Part model, mm, in its own coordinate system. A direction names the side the tool comes from. Coordinates: 2 decimals unless noted, no trailing zeros. Loops run counter-clockwise (first coordinate to the right, second up) from the corner with the lowest first, then second, coordinate; pieces in that order, holes last. Notation, with made-up numbers: M 29.25,-30 L 82.25,-30 A7 cw 82.25,-23 Z; hole C 48.5,-15 d10. An arc over 180 degrees is marked long. Use a Markdown table: item, result. Add a question column.
1) Pull direction Y, two halves, no side cores. Call faces 1 (the flat face through (8, 0, 6.35)), 2 (the cylindrical face through (0.53, 16.36, 3.22)), 3 (the cylindrical face through (3.46, -6.016, 12.789)): released by +Y, released by -Y, zero draft, split by the parting line, or undercut.
2) Band-saw the part on B-B (y = 0). List the corners of the cut face in (x, z).
3) Band-saw the part on C-C (z = 16). List the corners of the cut face in (x, y) (1 decimal), plus the area to 3 significant figures.
4) Band-saw the part on D-D (x = 6). List the corners of the cut face in (y, z).
5) Tool access for faces 4 (the cylindrical face through (6.94, -0.01, 12.79)), 5 (the flat face through (-5.408, -3.079, 12.611)), 6 (the cylindrical face through (3.48, 6.004, 12.789)), 7 (the cylindrical face through (-6.94, 0.01, 12.79)): list every direction of +Z, -Z, +X, -X, +Y, -Y with a clear straight run to the whole face (end or side of a thin tool).
6) Wall check: probe 1 along Y at (x, z) = (0, 5.25); probe 2 along Z at (x, y) = (-8.5, 2); probe 3 along Y at (x, z) = (13.5, 4.5). Give the ranges that are in metal, low to high. Write a range as from..to.
7) Pin check, flat tips, straight feed: pin 1 Ø1.7 at (x, y) = (0, 15.08) entering from +Z; pin 2 Ø2.5 at (x, z) = (-1, 9.5) entering from +Y; pin 3 Ø10 at (y, z) = (1.5, 12) entering from -X; pin 4 Ø1 at (x, z) = (5.5, 8.5) entering from +Y. Stop position of each tip, or through.
8) Band-saw the part on A-A (x = 0). List the corners of the cut face in (y, z).
Autodesk Fusion 360 part; units mm, degrees
sketch "Sketch1" plane through (0, 0, 0) normal (0, 0, 1) x (1, 0, 0)
  circle A0 centre (0, 0) radius 18.2563
  circle A1 centre (0, 0) radius 15.0812 construction
  line L0 (0, 0) -> (0, 18.2563) construction
  line L1 (3.5929, -6.223) -> (7.1857, 0)
  line L2 (7.1857, 0) -> (3.5929, 6.223)
  line L3 (3.5929, 6.223) -> (-3.5929, 6.223)
  line L4 (-3.5929, 6.223) -> (-7.1857, 0)
  line L5 (-7.1857, 0) -> (-3.5929, -6.223)
  line L6 (-3.5929, -6.223) -> (3.5929, -6.223)
  point P0 (0, 15.0812)
  dimension "d1" = 36.5125
  dimension "d2" = 30.1625
  dimension "d3" = 6.223
extrude "Extrude1" add sketch "Sketch1" along normal blind 6.35
extrude "Extrude2" add sketch "Sketch1" along normal blind 19.05 contours L1 L2 L3 L4 L5 L6
hole "Hole1" at (0, 15.0812, 0) direction (0, 0, 1) diameter 2.7686 depth 6.35 tip angle 118
pattern_circular "C-Pattern1" count 3 over 360 about axis through (0, 0, 0) along (0, 0, 1) of "Hole1"
fillet "Fillet1" radius 1.5875 6 edges at (3.5929, -6.223, 12.7) (-3.5929, -6.223, 12.7) (-7.1857, 0, 12.7) (-3.5929, 6.223, 12.7) (3.5929, 6.223, 12.7) (7.1857, 0, 12.7)
equation "d6 = d4 + shankLength"
equation "d14 = ( 1 / 16 ) * 1 in"
equation "shankLength = 0.5 in"
Entries:
| question | item | result |
|---|---|---|
| 1 | face 1 | zero draft |
| 1 | face 2 | undercut |
| 1 | face 3 | released by -Y |
| 2 | outline | M -18.26,0 L 18.26,0 L 18.26,6.35 L 6.94,6.35 L 6.94,19.05 L -6.94,19.05 L -6.94,6.35 L -18.26,6.35 Z |
| 3 | outline | M -6.7,-0.8 L -4.1,-5.4 A1.6 ccw -2.7,-6.2 L 2.7,-6.2 A1.6 ccw 4.1,-5.4 L 6.7,-0.8 A1.6 ccw 6.7,0.8 L 4.1,5.4 A1.6 ccw 2.7,6.2 L -2.7,6.2 A1.6 ccw -4.1,5.4 L -6.7,0.8 A1.6 ccw Z |
| 3 | area | 133 mm2 |
| 4 | outline | M -17.24,0 L 17.24,0 L 17.24,6.35 L 2.05,6.35 L 2.05,19.05 L -2.05,19.05 L -2.05,6.35 L -17.24,6.35 Z |
| 5 | face 4 | +Z, +X |
| 5 | face 5 | +Z, -X, -Y |
| 5 | face 6 | +Z, +X, +Y |
| 5 | face 7 | +Z, -X |
| 6 | probe 1 | -18.26..13.7, 16.47..18.26 |
| 6 | probe 2 | 0..6.35 |
| 6 | probe 3 | -12.29..-8.85, -6.23..12.29 |
| 7 | pin 1 | through |
| 7 | pin 2 | y = 6.22 |
| 7 | pin 3 | x = -6.94 |
| 7 | pin 4 | y = 3.79 |
| 8 | outline | M -18.26,0 L 13.7,0 L 13.7,6.35 L 6.22,6.35 L 6.22,19.05 L -6.22,19.05 L -6.22,6.35 L -18.26,6.35 Z; M 16.47,0 L 18.26,0 L 18.26,6.35 L 16.47,6.35 Z |
